```python
from build123d import *

# Parameters (mm, degrees)
F0_W     = 24
F0_H     = 70
F1_DEPTH = 24
F2_T     = -2
F3_R     = 2.85
F4_DEPTH = 3


with BuildPart() as f1:
    # F0 (on Front) → F1 (new body)
    with BuildSketch(Plane.XZ):
        with Locations((12, 35)):
            Rectangle(F0_W, F0_H)
    extrude(amount=F1_DEPTH)

    # F2
    f2_openings = [f1.faces().sort_by_distance(p)[0] for p in [
        (12, -12, 70),
        (12, -12, 0),
    ]]
    offset(amount=F2_T, openings=f2_openings)

    # F3 (on Front) → F4 (cut)
    with BuildSketch(Plane.XZ):
        with Locations((12, 57.445619)):
            Circle(F3_R)
    extrude(amount=F4_DEPTH, mode=Mode.SUBTRACT)


solid = f1.part
```
Build history of the part. All positions in model axes, mm. A direction names the side the tool comes from. Coordinates: 2 decimals unless noted, no trailing zeros. Order: outer loops, then holes, each group sorted by start corner. A loop starts at its lowest first (then second) coordinate and runs counter-clockwise, first axis right, second up. Notation, with made-up numbers: (-19.75, 62.5) -> (-13.75, 62.5) arc R16 ccw to (-13.75, 76.5) -> close; hole circle Ø8 at (64.25, 26.25). An arc over 180 degrees is marked (long way). Answer in a Markdown table with one row per item. Add a question column.
Q1. Drop a flat-ended pin along its axis: pin 1 (5 mm diameter, centred on y = -12.5, z = 15, fed in from -X). Give the stop position or say it passes through.
Q2. Band-saw the part on B-B, the plane y = -18. List the corners of the cut face in (x, z).
Q3. Which spindle directions (+Z, -Z, +X, -X, +Y, -Y) get a long thin tool onto all of the face, cutting with end or side? Do faces 1 (the face through (12, -22, 35)), 2 (the face through (22.5, -11.8, 70)), 3 (the face through (9.9, -0.99, 59.37)). Say none if no direction does.
Q4. Band-saw the part on C-C, the plane x = 5.5. List the corners of the cut face in (y, z), then the cut area to 3 significant figures.
Q5. Band-saw the part on A-A, the plane x = 12. List the corners of the cut face in (y, z).
Q6. Mould opens along X. For faces 4 (the face through (12, -24, 35)), 5 (the face through (22, -12, 35)), 6 (the face through (24, -12, 35)), 7 (the face through (0, -12, 35)) say: +X half, -X half, draft (parallel to the pull), parting line (faces both ways), or undercut.
Q7. Wall check: line 1 along X through (y, z) = (-19, 17.5); line 2 along Y through (x, z) = (16.25, 12); line 3 along Z through (x, y) = (12, -1). Give the ranges that are in metal, low to high. Write a range as [from, to].
Q8. Band-saw the part on D-D, the plane z = 61.5. List the corners of the cut face in (x, y).
Answers follow:
| question | item | result |
|---|---|---|
| 1 | pin 1 | x = 0 |
| 2 | outline | (0, 0) -> (2, 0) -> (2, 70) -> (0, 70) -> close; (22, 0) -> (24, 0) -> (24, 70) -> (22, 70) -> close |
| 3 | face 1 | +Z, -Z |
| 3 | face 2 | +Z, +X, -X, +Y, -Y |
| 3 | face 3 | +Y |
| 4 | outline | (-24, 0) -> (-22, 0) -> (-22, 70) -> (-24, 70) -> close; (-2, 0) -> (0, 0) -> (0, 70) -> (-2, 70) -> close |
| 4 | area | 280 mm^2 |
| 5 | outline | (-24, 0) -> (-22, 0) -> (-22, 70) -> (-24, 70) -> close; (-2, 0) -> (0, 0) -> (0, 54.6) -> (-2, 54.6) -> close; (-2, 60.3) -> (0, 60.3) -> (0, 70) -> (-2, 70) -> close |
| 6 | face 4 | draft |
| 6 | face 5 | undercut |
| 6 | face 6 | +X half |
| 6 | face 7 | -X half |
| 7 | line 1 | [0, 2], [22, 24] |
| 7 | line 2 | [-24, -22], [-2, 0] |
| 7 | line 3 | [0, 54.6], [60.3, 70] |
| 8 | outline | (0, -24) -> (24, -24) -> (24, 0) -> (0, 0) -> close; hole (2, -22) -> (22, -22) -> (22, -2) -> (2, -2) -> close |
